The model under review builds one solid part; all positions refer to its coordinate system, in mm. A direction names the side the tool comes from. Coordinates: 2 decimals unless noted, no trailing zeros. Loops run counter-clockwise (first coordinate to the right, second up) from the corner with the lowest first, then second, coordinate; pieces in that order, holes last. Notation, with made-up numbers: M 62,38.25 L 120,38.25 A11 ccw 120,55.25 Z; hole C 9,-28.75 d10. An arc over 180 degrees is marked long. Write item = value, one per line. Start each with the question number.
Q1. Wall thickness on probe 1 along Y at (x, z) = (-3.5, 0); probe 2 along Y at (x, z) = (6.55, 0); probe 3 along X at (y, z) = (-1.5, -1): over which ranges is each line inside the solid? List them lowest first.
Q2. Clearance check with flat-ended pins moving along their axes: pin 1 Ø0.6 at (y, z) = (-0.5, -3.5) entering from +X; pin 2 Ø0.9 at (x, z) = (4.5, 3) entering from -Y; pin 3 Ø2.5 at (x, z) = (6.5, 3) entering from +Y. State where each tip first meets the part, or that it passes through.
Q3. We need section B-B on z = 0. Give the boundary of the cut face in (x, y), and give its area (3 significant figures).
Q4. Mouldability with a two-part tool opening along Y and no side actions: class faces 5 (the face through (-1.972, 1.978, 2.579)), 6 (the face through (8, -3, 0)), 7 (the face through (6, 1, 3)) as released by +Y, released by -Y, zero draft, split by the parting line, or undercut.
Q5. For faces 1 (the face through (-4, -2.8, -1)), 2 (the face through (-6.028, 2.144, -1.824)), 3 (the face through (6, -1, -3)), 4 (the face through (-6.028, -2.144, 1.824)), list the 3-axis set-ups (+Z, -Z, +X, -X, +Y, -Y) from which the entire face can be reached by the end or side of a thin tool; tool diameter is ignored.
Q6. We need section C-C on x = 4.75. Give the boundary of the cut face in (y, z).
Q7. We need section D-D on y = 0. Give the boundary of the cut face in (x, z).
Q8. We need section A-A on x = -4.75. Give the boundary of the cut face in (y, z), and give its area (3 significant figures).
from build123d import *

# Parameters (mm, degrees)
SKETCH_1_R          = 4.8
SKETCH_1_R_2        = 2
EXTRUDE_1_DEPTH     = 8
SKETCH_2_W          = 12
SKETCH_2_H          = 2
CUT_EXTRUDE_1_DEPTH = 5
SKETCH_7_R          = 2
EXTRUDE_4_DEPTH     = 2
SKETCH_8_R          = 3.25
EXTRUDE_5_DEPTH     = 8
SKETCH_9_R          = 1.35
CUT_EXTRUDE_3_DEPTH = 18.380448786
SKETCH_10_OUTSIDE_W = 15.796
SKETCH_10_OUTSIDE_H = 15.796
CUT_EXTRUDE_4_DEPTH = 4


with BuildPart() as part:
    # 草图1 → 凸台-拉伸1 (new body)
    with BuildSketch(Plane(origin=(0, 0, 0), x_dir=(0, 0, -1), z_dir=(1, 0, 0))):
        Circle(SKETCH_1_R)
        Circle(SKETCH_1_R_2, mode=Mode.SUBTRACT)
    extrude(amount=EXTRUDE_1_DEPTH)

    # 草图2 → 切除-拉伸1 (cut)
    with BuildSketch(Plane(origin=(8, 0, 0), x_dir=(0, 0, -1), z_dir=(1, 0, 0))):
        with Locations((0.025285626, 0)):
            Rectangle(SKETCH_2_W, SKETCH_2_H)
    extrude(amount=-CUT_EXTRUDE_1_DEPTH, mode=Mode.SUBTRACT)

    # 草图7 → 凸台-拉伸4 (add)
    with BuildSketch(Plane.ZY):
        Circle(SKETCH_7_R)
    extrude(amount=-EXTRUDE_4_DEPTH)

    # 草图8 → 凸台-拉伸5 (add)
    with BuildSketch(Plane.ZY):
        with Locations(Location((0, 0, 0), (0, 0, 180))):
            Circle(SKETCH_8_R)
    extrude(amount=EXTRUDE_5_DEPTH)

    # 草图9 → 切除-拉伸3 (cut, through all)
    with BuildSketch(Plane.ZY.offset(8)):
        Circle(SKETCH_9_R)
    extrude(amount=-CUT_EXTRUDE_3_DEPTH, mode=Mode.SUBTRACT)

    # 草图10 outside → 切除-拉伸4 (cut)
    with BuildSketch(Plane.ZY.offset(8)):
        Rectangle(SKETCH_10_OUTSIDE_W, SKETCH_10_OUTSIDE_H)
        Polygon((-3.070099371, 1.066297262), (-2.458490203, -2.125635416), (0.611609168, -3.191932679), (3.070099371, -1.066297262), (2.458490203, 2.125635416), (-0.611609168, 3.191932679), align=None, mode=Mode.SUBTRACT)
    extrude(amount=-CUT_EXTRUDE_4_DEPTH, mode=Mode.SUBTRACT)


solid = part.part
Returned:
q1.probe_1 = -3.25 to -1.35, 1.35 to 3.25
q1.probe_2 = -4.8 to -2, 2 to 4.8
q1.probe_3 = -8 to 2
q2.pin_1 = 3
q2.pin_2 = -4.07
q2.pin_3 = 4.47
q3.outline = M -8,-2.98 L -4,-2.98 L -4,-3.25 L 0,-3.25 L 0,-4.8 L 8,-4.8 L 8,-2 L 2,-2 L 2,-1.35 L -8,-1.35 Z; M -8,1.35 L 2,1.35 L 2,2 L 8,2 L 8,4.8 L 0,4.8 L 0,3.25 L -4,3.25 L -4,2.98 L -8,2.98 Z
q3.area = 75.6 mm^2
q4.face_5 = split by the parting line
q4.face_6 = zero draft
q4.face_7 = undercut
q5.face_1 = -Z, -X, -Y
q5.face_2 = -Z, -X, +Y
q5.face_3 = +Z, -Z, +X
q5.face_4 = +Z, -X, -Y
q6.outline = M -1,-4.69 L -1,-1.73 A2 cw -1,1.73 L -1,4.69 A4.8 ccw Z; M 1,-4.69 A4.8 ccw 1,4.69 L 1,1.73 A2 cw 1,-1.73 Z
q7.outline = M -8,-2.87 L -4,-2.87 L -4,-3.25 L 0,-3.25 L 0,-4.8 L 3,-4.8 L 3,-2 L 2,-2 L 2,-1.35 L -8,-1.35 Z; M -8,1.35 L 2,1.35 L 2,2 L 3,2 L 3,4.8 L 0,4.8 L 0,3.25 L -4,3.25 L -4,2.87 L -8,2.87 Z
q8.outline = M -3.19,0.61 L -2.13,-2.46 L 1.07,-3.07 L 3.19,-0.61 L 2.13,2.46 L -1.07,3.07 Z; hole C 0,0 d2.7
q8.area = 21.7 mm^2
